Autodesk Inventor part; units mm, degrees
ref_plane "YZ Plane" through (0, 0, 0) normal (1, 0, 0) x (0, 1, 0)
ref_plane "XZ Plane" through (0, 0, 0) normal (0, 1, 0) x (-1, 0, 0)
ref_plane "XY Plane" through (0, 0, 0) normal (0, 0, 1) x (1, 0, 0)
sketch "Sketch1" plane through (0, 0, 0) normal (1, 0, 0) x (0, 1, 0)
  circle A0 centre (0, 0) radius 7.112
  circle A1 centre (0, 0) radius 12.7
  line L0 (10.8193, 6.6508) -> (10.8193, -6.6508)
  line L1 (-0.3501, 12.6952) -> (11.1694, 6.0444)
  line L2 (-11.1694, 6.0444) -> (0.3501, 12.6952)
  line L3 (-10.8193, -6.6508) -> (-10.8193, 6.6508)
  line L4 (0.3501, -12.6952) -> (-11.1694, -6.0444)
  line L5 (11.1694, -6.0444) -> (-0.3501, -12.6952)
  point P0 (0, -12.4931)
  point P1 (10.8193, -6.2465)
  point P2 (10.8193, 6.2465)
  point P3 (0, 12.4931)
  point P4 (-10.8193, 6.2465)
  point P5 (-10.8193, -6.2465)
  dimension "d0" = 14.224
  dimension "d1" = 25.4
  dimension "d6" = 360
extrude "Extrusion2" add sketch "Sketch1" along normal blind 3.048 contours L0 L5 L4 L3 L2 L1
properties part number "CH-2(Gearbox_Output_Spacer)"
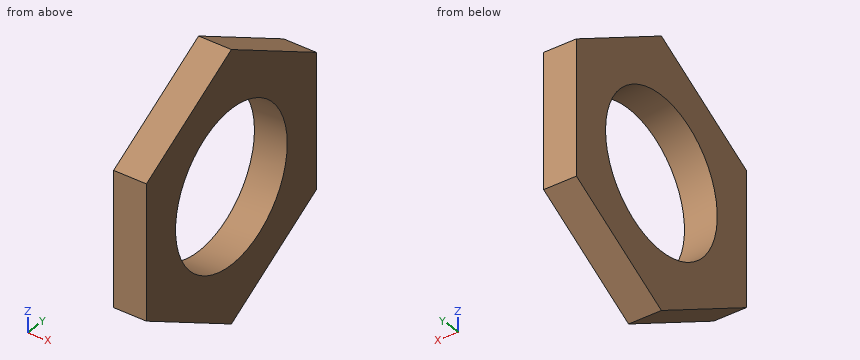
Geometry: final body of the model. Coordinates: model frame, mm. Coordinates: 2 decimals unless noted, no trailing zeros. Write each loop counter-clockwise with the first axis right and the second up, starting at its lowest first coordinate (ties: lowest second). Pieces come first, ordered by that corner, then holes. Notation, with made-up numbers: (12.25, 38.5) - (33.25, 38.5) arc R21 cw to (33.25, 74.5) - close; hole circle Ø9 at (-37, -19). An arc over 180 degrees is marked (long way). Return JSON: item names as keys, results as strings.
Item 1: Section query D-D (z = 7.75). Output: boundary loops of the cut face in (x, y), and give its area (3 significant figures).
Completed:
{"outline": "(0, -8.22) - (3.05, -8.22) - (3.05, 8.22) - (0, 8.22) - close", "area": "50.1 mm2"}
Item 2: Section query A-A (x = 2.1). Output: boundary loops of the cut face in (y, z).
Completed:
{"outline": "(-10.82, -6.25) - (0, -12.49) - (10.82, -6.25) - (10.82, 6.25) - (0, 12.49) - (-10.82, 6.25) - close; hole circle Ø14.22 at (0, 0)"}
Item 3: Section query C-C (y = 1.5). Output: boundary loops of the cut face in (x, z).
Completed:
{"outline": "(0, -11.63) - (3.05, -11.63) - (3.05, -6.95) - (0, -6.95) - close; (0, 6.95) - (3.05, 6.95) - (3.05, 11.63) - (0, 11.63) - close"}
Item 4: Section query B-B (z = 0). Output: boundary loops of the cut face in (x, y), and give its area (3 significant figures).
Completed:
{"outline": "(0, -10.82) - (3.05, -10.82) - (3.05, -7.11) - (0, -7.11) - close; (0, 7.11) - (3.05, 7.11) - (3.05, 10.82) - (0, 10.82) - close", "area": "22.6 mm2"}
Item 5: Line query: L1, parallel to Z at x = 1.8, y = -6; L2, parallel to Y at x = 0.6, z = 6.5; L3, parallel to Y at x = 0.4, z = 2.5. Output: solid intervals per line, ascending.
Completed:
{"L1": "z = -9.03 to -3.82, 3.82 to 9.03", "L2": "y = -10.38 to -2.89, 2.89 to 10.38", "L3": "y = -10.82 to -6.66, 6.66 to 10.82"}
